Here's the drawing with two shaded views (mm, measured from the low corner). I have some questions. A direction names the side the tool comes from. Round coordinates to 2 decimals unless told otherwise and drop trailing zeros. Order: outer loops, then holes, each group sorted by start corner. A loop starts at its lowest first (then second) coordinate and runs counter-clockwise, first axis right, second up. Notation, with made-up numbers: (-38.5, 46) -> (11.5, 46) arc R26 cw to (11.5, 69) -> close; hole circle Ø8 at (85.25, 84). An arc over 180 degrees is marked (long way). Answer in a Markdown table with one row per item.
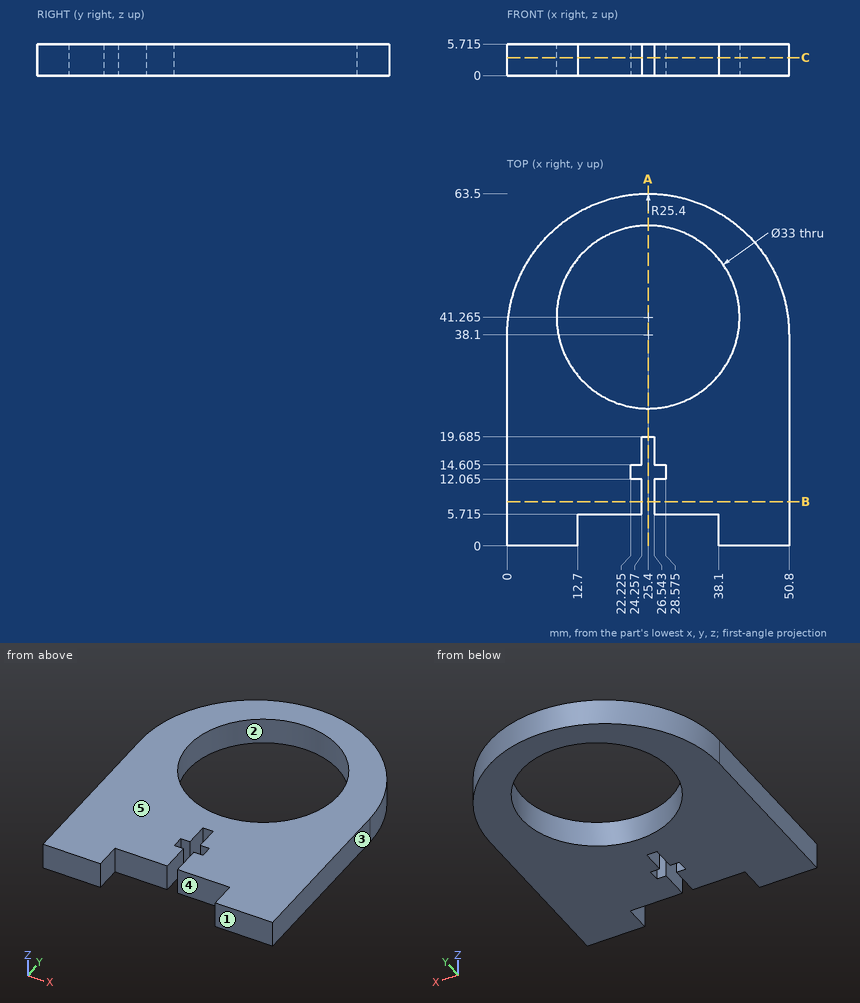
1. Please list where these lines run through material, in increasing order: line 1 along Y through (x, z) = (25.4, 2.3) (3 decimals); line 2 along X through (y, z) = (8, 4.15); line 3 along Y through (x, z) = (22.5, 4) (1 decimal).
Numbers:
| item | result |
|---|---|
| line 1 | y = 19.685 to 24.765, 57.765 to 63.5 |
| line 2 | x = 0 to 24.26, 26.54 to 50.8 |
| line 3 | y = 5.7 to 12.1, 14.6 to 25, 57.5 to 63.3 |
2. Suppose I cut it at A-A on x = 25.4. Write out the boundary of the cut face in (y, z) (3 decimals), then the cut area to 3 significant figures.
Numbers:
| item | result |
|---|---|
| outline | (19.685, 0) -> (24.765, 0) -> (24.765, 5.715) -> (19.685, 5.715) -> close; (57.765, 0) -> (63.5, 0) -> (63.5, 5.715) -> (57.765, 5.715) -> close |
| area | 61.8 mm2 |
3. For pin 1 Ø2 at (y, z) = (18.5, 4.5) entering from -X; pin 2 Ø0.6 at (x, z) = (23.5, 3.5) entering from +Y; pin 3 Ø2.5 at (x, z) = (25, 2.5) entering from -Y (3 decimals); pin 4 Ø2 at (x, z) = (32.5, 4.5) entering from +Y, each with a flat end and sliding along its axis, tell me the tip position at first contact or that it passes through.
Numbers:
| item | result |
|---|---|
| pin 1 | stops at x = 0 |
| pin 2 | stops at y = 63.45 |
| pin 3 | stops at y = 5.715 |
| pin 4 | stops at y = 62.76 |
4. Suppose I cut it at B-B on y = 8. Write out the boundary of the cut face in (x, z) (3 decimals).
Numbers:
| item | result |
|---|---|
| outline | (0, 0) -> (24.257, 0) -> (24.257, 5.715) -> (0, 5.715) -> close; (26.543, 0) -> (50.8, 0) -> (50.8, 5.715) -> (26.543, 5.715) -> close |
5. Suppose I cut it at C-C on z = 3.25. Write out the boundary of the cut face in (x, y) (3 decimals), then the cut area to 3 significant figures.
Numbers:
| item | result |
|---|---|
| outline | (0, 0) -> (12.7, 0) -> (12.7, 5.715) -> (24.257, 5.715) -> (24.257, 12.065) -> (22.225, 12.065) -> (22.225, 14.605) -> (24.257, 14.605) -> (24.257, 19.685) -> (26.543, 19.685) -> (26.543, 14.605) -> (28.575, 14.605) -> (28.575, 12.065) -> (26.543, 12.065) -> (26.543, 5.715) -> (38.1, 5.715) -> (38.1, 0) -> (50.8, 0) -> (50.8, 38.1) arc R25.4 ccw to (0, 38.1) -> close; hole circle Ø33 at (25.4, 41.265) |
| area | 1,910 mm2 |
6. We'd pull the mould along Y, two halves only. Please class the marked faces 1, 2 and 3: released by +Y, released by -Y, zero draft, split by the parting line, or undercut.
Numbers:
| item | result |
|---|---|
| face 1 | released by -Y |
| face 2 | undercut |
| face 3 | zero draft |
7. For the marked faces 4 and 5, which set-ups out of +Z, -Z, +X, -X, +Y, -Y let a thin tool reach every point of the face, with its end or its side?
Numbers:
| item | result |
|---|---|
| face 4 | +Z, -Z, -Y |
| face 5 | +Z, +X, -X, +Y, -Y |
